Could you check a few things on this model? Use its own coordinates, in mm. Give positions to 0.01 mm unless a question says otherwise; leave off trailing zeros. Loops run counter-clockwise (first coordinate to the right, second up) from the corner with the lowest first, then second, coordinate; pieces in that order, holes last. Notation, with made-up numbers: (-6, 60) -> (44, 60) arc R23 cw to (44, 80) -> close; hole circle Ø1 at (13, 16.5). An arc over 180 degrees is marked (long way). Write each question's results on one line, items separated by ' | '. Start each with the question number.
Q1. Will these pins go through, and if not, where does the flat tip stop? P1, Ø0.9, axis at x = 108, y = 1.5, coming from the -Z side; P2, Ø0.9, axis at x = 1.5, y = 1, coming from the +Z side; P3, Ø1.5, axis at y = 1.5, z = -235.5, coming from the -X side.
Q2. If we section it at B-B, the plane x = 125.5: List the corners of the cut face in (y, z) for me, plus the area to 3 significant figures.
Q3. If I drill on line 1 along Z through (x, y) = (13.5, 1.2); line 2 along X through (y, z) = (1.35, -152); line 3 along X through (y, z) = (2, -112), over which ranges is the centre line in solid material (lowest first)?
Q4. If we section it at A-A, the plane z = -150: List the corners of the cut face in (x, y) for me, plus the area to 3 significant figures.
from build123d import *

# Parameters (mm, degrees)
SALIENTE_EXTRUIR1_DEPTH = 3


with BuildPart() as part:
    # Croquis1 → Saliente-Extruir1 (new body)
    with BuildSketch(Plane(origin=(0, 0, 0), x_dir=(1, 0, 0), z_dir=(0, 1, 0))):
        Polygon((17.5, 0), (32.5, 0), (32.5, 3), (47.5, 3), (47.5, 0), (62.5, 0), (62.5, 3), (77.5, 3), (77.5, 0), (92.5, 0), (92.5, 3), (110, 3), (110, 10), (107, 10), (107, 25), (110, 25), (110, 40), (107, 40), (107, 55), (110, 55), (110, 65), (107, 65), (107, 68), (117.5, 68), (117.5, 65), (132.5, 65), (132.5, 68), (147.5, 68), (147.5, 65), (162.5, 65), (162.5, 68), (177.5, 68), (177.5, 65), (192.5, 65), (192.5, 68), (207.5, 68), (207.5, 65), (222.5, 65), (222.5, 68), (237.5, 68), (237.5, 65), (252.5, 65), (252.5, 68), (260, 68), (260, 82.5), (257, 82.5), (257, 97.5), (260, 97.5), (260, 112.5), (257, 112.5), (257, 127.5), (260, 127.5), (260, 142.5), (257, 142.5), (257, 157.5), (260, 157.5), (260, 172.5), (257, 172.5), (257, 187.5), (260, 187.5), (260, 202.5), (257, 202.5), (257, 217.5), (260, 217.5), (260, 232.5), (257, 232.5), (257, 247.5), (260, 247.5), (260, 265), (242.5, 265), (242.5, 262), (227.5, 262), (227.5, 265), (212.5, 265), (212.5, 262), (197.5, 262), (197.5, 265), (182.5, 265), (182.5, 262), (167.5, 262), (167.5, 265), (152.5, 265), (152.5, 262), (137.5, 262), (137.5, 265), (122.5, 265), (122.5, 262), (107.5, 262), (107.5, 265), (92.5, 265), (92.5, 262), (77.5, 262), (77.5, 265), (62.5, 265), (62.5, 262), (47.5, 262), (47.5, 265), (32.5, 265), (32.5, 262), (17.5, 262), (17.5, 265), (0, 265), (0, 245), (3, 245), (3, 230), (0, 230), (0, 215), (3, 215), (3, 200), (0, 200), (0, 185), (3, 185), (3, 170), (0, 170), (0, 155), (3, 155), (3, 140), (0, 140), (0, 125), (3, 125), (3, 110), (0, 110), (0, 95), (3, 95), (3, 80), (0, 80), (0, 62), (3, 62), (3, 50), (0, 50), (0, 35), (3, 35), (3, 20), (0, 20), (0, 3), (17.5, 3), align=None)
    extrude(amount=SALIENTE_EXTRUIR1_DEPTH)


solid = part.part
Final values:
1) P1: stops at z = -262 | P2: stops at z = -3 | P3: stops at x = 3
2) outline: (0, -265) -> (3, -265) -> (3, -65) -> (0, -65) -> close | area: 600 mm²
3) line 1: z = -265 to -3 | line 2: x = 3 to 257 | line 3: x = 3 to 260
4) outline: (3, 0) -> (257, 0) -> (257, 3) -> (3, 3) -> close | area: 762 mm²
